Autodesk Inventor part; units mm, degrees
ref_plane "YZ Plane" through (0, 0, 0) normal (1, 0, 0) x (0, 1, 0)
ref_plane "XZ Plane" through (0, 0, 0) normal (0, 1, 0) x (-1, 0, 0)
ref_plane "XY Plane" through (0, 0, 0) normal (0, 0, 1) x (1, 0, 0)
sketch "Sketch1" plane through (0, 0, 0) normal (0, 0, 1) x (1, 0, 0)
  line L0 (0, 0) -> (0, 152.4)
  line L1 (0, 152.4) -> (1.524, 152.4)
  line L2 (25.4, 128.524) -> (25.4, 38.1)
  line L3 (0, 0) -> (152.4, 0)
  line L4 (152.4, 0) -> (152.4, 1.524)
  line L5 (128.524, 25.4) -> (38.1, 25.4)
  arc A0 (25.4, 38.1) -> (38.1, 25.4) centre (38.1, 38.1) ccw
  arc A1 (25.4, 128.524) -> (1.524, 152.4) centre (1.524, 128.524) ccw
  arc A2 (152.4, 1.524) -> (128.524, 25.4) centre (128.524, 1.524) ccw
  line L6 (0, 188.8139) -> (0, -31.469)
  line L7 (-31.469, 0) -> (188.8139, 0)
  point P0 (0, 0)
  dimension "thickness" = 25.4
  dimension "d3" = 25.4
  dimension "LegSize" = 152.4
  dimension "d5" = 152.4
  dimension "radius" = 12.7
  dimension "d7" = 23.876
  dimension "d8" = 23.876
  dimension "d11" = 0
  dimension "d12" = 0
extrude "6\" X 6\" X 1\"" add sketch "Sketch1" along normal mid plane 300
equation "\"d3\" = thickness"
equation "\"d5\" = LegSize"
properties part number "ANGLE IRON, 6 X 6 X 1 THK" material "Angle Iron"
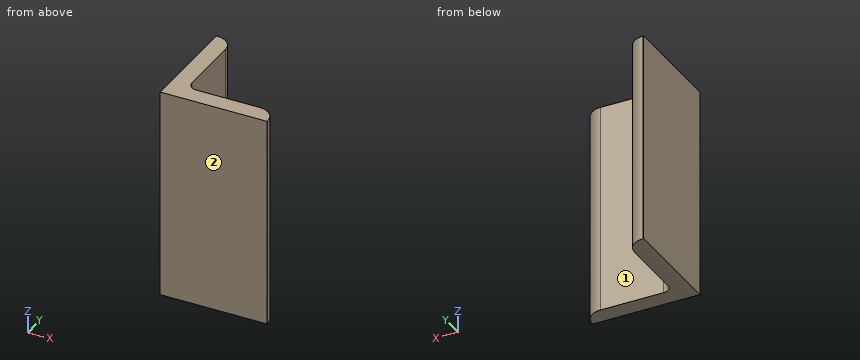
The listing builds one solid part. Answer for the finished solid, in the listing's coordinates (mm). Face numbers are marked on the shaded views. A direction names the side the tool comes from. Round coordinates to 2 decimals unless told otherwise and drop trailing zeros. Loops run counter-clockwise (first coordinate to the right, second up) from the corner with the lowest first, then second, coordinate; pieces in that order, holes last.
Q1. Section B-B, the plane y = 81.5 is taken. Determine the outline of the cut face in (x, z), then the cut area to 3 significant figures.
Q2. Find the intervals of material crossed by line 1 (Y direction, x = 44, z = -121.5); line 2 (X direction, y = 141, z = -22.5), in increasing order.
Q3. Section A-A, the plane z = -36 is taken. Determine the outline of the cut face in (x, y), then the cut area to 3 significant figures.
Q4. Given pin 1 Ø4 at (x, z) = (29.5, 107.5) entering from +Y (3 decimals); pin 2 Ø1 at (x, z) = (100.5, -11) entering from +Y; pin 3 Ø6 at (y, z) = (59, 37.5) entering from +X, each flat-ended and moving along its own axis, determine where each tip first touches the part or whether it passes through.
Q5. Which of the six approach directions +Z, -Z, +X, -X, +Y, -Y give full straight-line access (tool end or side, diameter ignored) to the marked faces 1 and 2?
Completed:
1. outline: (0, -150) - (25.4, -150) - (25.4, 150) - (0, 150) - close
1. area: 7,620 mm2
2. line 1: y = 0 to 25.4
2. line 2: x = 0 to 21.88
3. outline: (0, 0) - (152.4, 0) - (152.4, 1.52) arc R23.88 ccw to (128.52, 25.4) - (38.1, 25.4) arc R12.7 cw to (25.4, 38.1) - (25.4, 128.52) arc R23.88 ccw to (1.52, 152.4) - (0, 152.4) - close
3. area: 6,890 mm2
4. pin 1: stops at y = 31.105
4. pin 2: stops at y = 25.4
4. pin 3: stops at x = 25.4
5. face 1: +Z, -Z, +X, +Y
5. face 2: +Z, -Z, +X, -X, -Y
